Design review of the part built by this model. Coordinates are the model's own, in mm. A direction names the side the tool comes from. Coordinates: 2 decimals unless noted, no trailing zeros. Order: outer loops, then holes, each group sorted by start corner. A loop starts at its lowest first (then second) coordinate and runs counter-clockwise, first axis right, second up.
Autodesk Inventor part; units mm, degrees
ref_plane "YZ Plane" through (0, 0, 0) normal (1, 0, 0) x (0, 1, 0)
ref_plane "XZ Plane" through (0, 0, 0) normal (0, 1, 0) x (-1, 0, 0)
ref_plane "XY Plane" through (0, 0, 0) normal (0, 0, 1) x (1, 0, 0)
sketch "Sketch1" plane through (0, 0, 0) normal (0, 1, 0) x (-1, 0, 0)
  line L0 (0, 0) -> (105, 0)
  line L1 (105, 0) -> (105, -50)
  line L2 (105, -50) -> (0, -50)
  line L3 (0, -50) -> (0, 0)
  line L4 (0, 0) -> (0, -16.6667)
  line L5 (0, -16.6667) -> (11, -16.6667)
  dimension "d0" = 105
  dimension "d1" = 50
  dimension "d2" = 16.6667
  dimension "d3" = 11
extrude "Extrusion1" add sketch "Sketch1" along normal blind 2
sketch "Sketch3" plane through (0, 2, 0) normal (0, 1, 0) x (1, 0, 0)
  circle A0 centre (-20, 12.5) radius 2.75
  line L0 (0, 0) -> (0, 50)
  line L1 (-105, 0) -> (0, 0)
  circle A1 centre (-20, 37.5) radius 2.75
  dimension "d21" = 5.5
  dimension "d22" = 20
  dimension "d23" = 12.5
  dimension "d26" = 25
extrude "Extrusion3" cut sketch "Sketch3" against normal through all
sketch "Sketch4" plane through (0, 2, 0) normal (0, 1, 0) x (1, 0, 0)
  circle A0 centre (-20, 12.5) radius 2.75
  line L0 (-20, 12.5) -> (-81, 12.5)
  line L1 (-81, 12.5) -> (-91, 12.5) construction
  line L2 (-81, 15.25) -> (-91, 15.25)
  line L3 (-91, 9.75) -> (-81, 9.75)
  arc A1 (-81, 9.75) -> (-81, 15.25) centre (-81, 12.5) ccw
  arc A2 (-91, 15.25) -> (-91, 9.75) centre (-91, 12.5) ccw
  point P0 (0, 0)
  point P1 (-86, 12.5)
  dimension "d33" = 61
  dimension "d34" = 10
  dimension "d35" = 5.5
extrude "Extrusion4" cut sketch "Sketch4" against normal through all contours A1 L3 A2 L2
pattern_linear "Rectangular Pattern2" count 2 spacing 25 along (0, 0, -1) of "Extrusion4"
sketch "Sketch5" plane through (0, 0, -50) normal (0, 0, -1) x (-1, 0, 0)
  line L0 (105, 0) -> (105, 2)
  line L1 (105, 0) -> (0, 0)
  line L2 (105, 2) -> (75, 2)
  line L3 (75, 2) -> (75, 0)
  line L4 (75, 0) -> (105, 0)
  line L5 (105, 0) -> (105, 2)
  dimension "d45" = 30
extrude "Extrusion5" add sketch "Sketch5" along normal blind 25
sketch "Sketch6" plane through (0, 2, 0) normal (0, 1, 0) x (1, 0, 0)
  line L0 (-85, 60.5) -> (-85, 70.5) construction
  line L1 (-82.25, 60.5) -> (-82.25, 70.5)
  line L2 (-87.75, 70.5) -> (-87.75, 60.5)
  arc A0 (-87.75, 60.5) -> (-82.25, 60.5) centre (-85, 60.5) ccw
  arc A1 (-82.25, 70.5) -> (-87.75, 70.5) centre (-85, 70.5) ccw
  line L3 (-75, 50) -> (-75, 75)
  arc A2 (-91, 40.25) -> (-91, 34.75) centre (-91, 37.5) ccw
  point P0 (0, 0)
  point P1 (-85, 65.5)
  dimension "d48" = 10
  dimension "d49" = 5.5
  dimension "d50" = 10
  dimension "d51" = 28
extrude "Extrusion6" cut sketch "Sketch6" against normal through all
fillet "Fillet2" radius 5 6 edges at (-105, 1, 0) (0, 1, 0) (-75, 1, -75) (-105, 1, -75) (0, 1, -50) (-75, 1, -50)
sketch "Sketch7" plane through (0, 2, 0) normal (0, 1, 0) x (1, 0, 0)
  circle A0 centre (-20, 12.5) radius 2.75
  line L0 (-20, 12.5) -> (-42, 12.5)
  line L1 (-42, 12.5) -> (-62, 12.5)
  circle A1 centre (-62, 12.5) radius 2.75
  circle A2 centre (-42, 12.5) radius 2.75
  line L2 (0, 5) -> (0, 45)
  line L3 (0, 0) -> (0, 45)
  circle A3 centre (-42, 37.5) radius 2.75
  circle A4 centre (-62, 37.5) radius 2.75
  dimension "d55" = 22
  dimension "d56" = 20
  dimension "d57" = 5.5
  dimension "d58" = 5.5
  dimension "d61" = 25
extrude "Extrusion7" cut sketch "Sketch7" against normal through all contours A1 | A2 L1 L0 | L0 L1 A2 | A3 | A4
sketch "Sketch9" plane through (0, 2, 0) normal (0, 1, 0) x (1, 0, 0)
  point P0 (0, 0)
sketch "Sketch10" plane through (0, 2, 0) normal (0, 1, 0) x (1, 0, 0)
  circle A0 centre (-100, 70) radius 2.75
  line L0 (-100, 75) -> (-80, 75)
  line L1 (-105, 5) -> (-105, 70)
  circle A1 centre (-100, 5) radius 2.75
  line L2 (-100, 0) -> (-5, 0)
  circle A2 centre (-5, 45) radius 2.75
  line L3 (-5, 50) -> (-70, 50)
  line L4 (0, 5) -> (0, 45)
  circle A3 centre (-5, 5) radius 2.75
  point P0 (0, 0)
  dimension "d70" = 5.5
  dimension "d71" = 5
  dimension "d72" = 5
  dimension "d73" = 5.5
  dimension "d74" = 5
  dimension "d75" = 5
  dimension "d76" = 5.5
  dimension "d77" = 5
  dimension "d78" = 5
  dimension "d79" = 5.5
  dimension "d80" = 5
  dimension "d81" = 5
extrude "Extrusion9" cut sketch "Sketch10" against normal through all
sketch "Sketch11" plane through (0, 2, 0) normal (0, 1, 0) x (1, 0, 0)
  circle A0 centre (-20, 37.5) radius 2.75
  line L0 (-20, 37.5) -> (-75, 37.5)
  line L1 (-75, 55) -> (-75, 70)
  line L2 (-75, 70) -> (-75, -9.6878)
  arc A1 (-75, 70) -> (-80, 75) centre (-80, 70) ccw
  line L3 (-75, 70) -> (-75, 84.2747)
  line L4 (-75, 84.2747) -> (39.8676, 84.2747)
  line L5 (39.8676, 84.2747) -> (39.8676, -9.6878)
  line L6 (39.8676, -9.6878) -> (-75, -9.6878)
  line L7 (-75, -9.6878) -> (-75, 84.2747)
  point P0 (0, 0)
  dimension "d86" = 55
extrude "Extrusion10" cut sketch "Sketch11" against normal through all
sketch "Sketch12" plane through (0, 2, 0) normal (0, 1, 0) x (1, 0, 0)
  line L0 (-108.4427, 0) -> (-97.25, 0)
  line L1 (-97.25, 0) -> (-97.25, 76.8209)
  line L2 (-97.25, 76.8209) -> (-108.4427, 76.8209)
  line L3 (-108.4427, 76.8209) -> (-108.4427, 0)
  point P0 (0, 0)
extrude "Extrusion11" cut sketch "Sketch12" against normal through all
fillet "Fillet3" radius 5 3 edges at (-97.25, 1, -75) (-97.25, 1, 0) (-75, 1, 0)
sketch "Sketch13" plane through (0, 2, 0) normal (0, 1, 0) x (1, 0, 0)
  arc A0 (-91, 40.25) -> (-91, 34.75) centre (-91, 37.5) ccw
  arc A1 (-81, 34.75) -> (-81, 40.25) centre (-81, 37.5) ccw
  line L0 (-91, 37.5) -> (-81, 37.5) construction
  line L1 (-91, 34.75) -> (-81, 34.75)
  line L2 (-81, 40.25) -> (-91, 40.25)
  arc A2 (-91, 40.25) -> (-91, 34.75) centre (-91, 37.5) ccw
  arc A3 (-81, 34.75) -> (-81, 40.25) centre (-81, 37.5) ccw
  arc A4 (-91, 15.25) -> (-91, 9.75) centre (-91, 12.5) ccw
  arc A5 (-81, 9.75) -> (-81, 15.25) centre (-81, 12.5) ccw
  line L3 (-91, 12.5) -> (-81, 12.5) construction
  line L4 (-91, 9.75) -> (-81, 9.75)
  line L5 (-81, 15.25) -> (-91, 15.25)
  arc A6 (-91, 15.25) -> (-91, 9.75) centre (-91, 12.5) ccw
  arc A7 (-81, 9.75) -> (-81, 15.25) centre (-81, 12.5) ccw
  line L6 (-91, 17.25) -> (-81, 17.25)
  arc A8 (-81, 7.75) -> (-81, 17.25) centre (-81, 12.5) ccw
  line L7 (-81, 7.75) -> (-91, 7.75)
  arc A9 (-91, 17.25) -> (-91, 7.75) centre (-91, 12.5) ccw
  line L8 (-91, 42.25) -> (-81, 42.25)
  arc A10 (-81, 32.75) -> (-81, 42.25) centre (-81, 37.5) ccw
  line L9 (-81, 32.75) -> (-91, 32.75)
  arc A11 (-91, 42.25) -> (-91, 32.75) centre (-91, 37.5) ccw
  arc A12 (-87.75, 60.5) -> (-82.25, 60.5) centre (-85, 60.5) ccw
  arc A13 (-82.25, 70.5) -> (-87.75, 70.5) centre (-85, 70.5) ccw
  line L10 (-85, 60.5) -> (-85, 70.5) construction
  line L11 (-87.75, 60.5) -> (-87.75, 70.5)
  line L12 (-82.25, 70.5) -> (-82.25, 60.5)
  arc A14 (-87.75, 60.5) -> (-82.25, 60.5) centre (-85, 60.5) ccw
  arc A15 (-82.25, 70.5) -> (-87.75, 70.5) centre (-85, 70.5) ccw
  line L13 (-80.25, 60.5) -> (-80.25, 70.5)
  arc A16 (-80.25, 70.5) -> (-89.75, 70.5) centre (-85, 70.5) ccw
  line L14 (-89.75, 70.5) -> (-89.75, 60.5)
  arc A17 (-89.75, 60.5) -> (-80.25, 60.5) centre (-85, 60.5) ccw
  point P0 (0, 0)
  point P1 (-86, 37.5)
  point P2 (-86, 12.5)
  point P3 (-85, 65.5)
  dimension "d92" = 2
  dimension "d93" = 2
  dimension "d94" = 2
extrude "Extrusion12" add sketch "Sketch13" along normal blind 1
properties part number "Belt_Restraint"
1. Add section D-D (x = -79.25). Give the boundary of the cut face in (y, z).
2. Add section C-C (x = -85). Give the boundary of the cut face in (y, z), and give its area (3 significant figures).
3. Add section A-A (z = -68). Give the boundary of the cut face in (x, y), and give its area (3 significant figures).
4. Mouldability with a two-part tool opening along Z and no side actions: class faces 5 (the cylindrical face through (-76, 1, -2)), 6 (the flat face through (-97.25, 1, -37)), 7 (the flat face through (-86, 1, -75)), 8 (the flat face through (-82.25, 2, -65)) as pulls with the +Z half, pulls with the -Z half, needs draft (parallel to the pull), parting line crosses it, or undercut.
5. Insertion check: pin 1 (1.5 mm diameter, centred on x = -88.5, y = 1.5, fed in from -Z). The pin has a flat end and moves straight along its axis. Give the tip position at first contact, or say it passes through.
6. To check wall thickness, follow line 1 (Z direction, x = -81, y = 1.4); line 2 (Z direction, x = -85, y = 0.3); line 3 (Y direction, x = -92.5, z = -56.5). State the ranges of each line that lie inside material, in increasing order.
7. Add section B-B (y = 1.45). Give the boundary of the cut face in (x, z).
8. For faces 1 (the cylindrical face through (-76.25, 2.49, -37.6)), 2 (the flat face through (-86, 2, -15.25)), 3 (the cylindrical face through (-84.9, 2.49, -55.75)), 4 (the cylindrical face through (-95.75, 2.49, -12.4)), list the 3-axis set-ups (+Z, -Z, +X, -X, +Y, -Y) from which the entire face can be reached by the end or side of a thin tool; tool diameter is ignored.
Solution:
1. outline: (0, -74.94) - (2, -74.94) - (2, -41.92) - (3, -41.92) - (3, -39.62) - (0, -39.62) - close; (0, -35.38) - (3, -35.38) - (3, -33.08) - (2, -33.08) - (2, -16.92) - (3, -16.92) - (3, -14.62) - (0, -14.62) - close; (0, -10.38) - (3, -10.38) - (3, -8.08) - (2, -8.08) - (2, -0.06) - (0, -0.06) - close
2. outline: (0, -75) - (2, -75) - (2, -75.25) - (3, -75.25) - (3, -73.25) - (0, -73.25) - close; (0, -57.75) - (3, -57.75) - (3, -55.75) - (2, -55.75) - (2, -42.25) - (3, -42.25) - (3, -40.25) - (0, -40.25) - close; (0, -34.75) - (3, -34.75) - (3, -32.75) - (2, -32.75) - (2, -17.25) - (3, -17.25) - (3, -15.25) - (0, -15.25) - close; (0, -9.75) - (3, -9.75) - (3, -7.75) - (2, -7.75) - (2, 0) - (0, 0) - close
2. area: 109 mm2
3. outline: (-97.25, 0) - (-87.75, 0) - (-87.75, 3) - (-89.75, 3) - (-89.75, 2) - (-97.25, 2) - close; (-82.25, 0) - (-75, 0) - (-75, 2) - (-80.25, 2) - (-80.25, 3) - (-82.25, 3) - close
3. area: 37.5 mm2
4. face 5: pulls with the +Z half
4. face 6: needs draft
4. face 7: pulls with the -Z half
4. face 8: undercut
5. pin 1: stops at z = -75
6. line 1: z = -75 to -40.25, -34.75 to -15.25, -9.75 to 0
6. line 2: z = -75 to -73.25, -57.75 to -40.25, -34.75 to -15.25, -9.75 to 0
6. line 3: y = 0 to 2
7. outline: (-97.25, -70) arc R5 ccw to (-92.25, -75) - (-80, -75) arc R5 ccw to (-75, -70) - (-75, -5) arc R5 ccw to (-80, 0) - (-92.25, 0) arc R5 ccw to (-97.25, -5) - close; hole (-91, -40.25) - (-81, -40.25) arc R2.75 ccw to (-81, -34.75) - (-91, -34.75) arc R2.75 ccw to start; hole (-91, -15.25) - (-81, -15.25) arc R2.75 ccw to (-81, -9.75) - (-91, -9.75) arc R2.75 ccw to start; hole (-87.75, -70.5) arc R2.75 ccw to (-82.25, -70.5) - (-82.25, -60.5) arc R2.75 ccw to (-87.75, -60.5) - close
8. face 1: +X, +Y
8. face 2: +Y, -Y
8. face 3: +Y
8. face 4: -X, +Y
